from build123d import *

# Parameters (mm, degrees)
BOSS_EXTRUDE1_DEPTH = 40
CUT_EXTRUDE1_DEPTH  = 25
CUT_EXTRUDE2_DEPTH  = 15
SKETCH3_R           = 2.5
CUT_EXTRUDE3_DEPTH  = 16
SKETCH3_6_R         = 6
SKETCH3_6_R_2       = 2.5
BOSS_EXTRUDE2_DEPTH = 10
FILLET2_R           = 2


with BuildPart() as part:
    # Sketch1 → Boss-Extrude1 (new body)
    with BuildSketch(Plane.XY):
        with BuildLine():
            Line((0, 0), (-50, 0))
            Line((-50, 0), (-50, -12.5))
            Line((-50, -12.5), (-60, -12.5))
            Line((-60, -12.5), (-60, -50.5))
            Line((-60, -50.5), (-46, -50.5))
            Line((-46, -50.5), (-33.311690981, -44.583344336))
            ThreePointArc((-33.311690981, -44.583344336), (-24.66100943, -43.235991833), (-16.596266659, -46.643274342))
            Line((-16.596266659, -46.643274342), (-12, -50.5))
            Line((-12, -50.5), (0, -50.5))
            Line((0, -50.5), (0, 0))
        make_face()
    extrude(amount=-BOSS_EXTRUDE1_DEPTH)

    # Sketch2 → Cut-Extrude1 (cut)
    with BuildSketch(Plane.XY):
        with BuildLine():
            ThreePointArc((-53.849159388, -20.384615385), (-51.013665761, -16.887003184), (-50, -12.5))
            Line((-50, -12.5), (-60, -12.5))
            Line((-60, -12.5), (-60, -22.5))
            ThreePointArc((-60, -22.5), (-56.747781822, -21.956377579), (-53.849159388, -20.384615385))
        make_face()
        with BuildLine():
            Line((0, 0), (-30, 0))
            ThreePointArc((-30, 0), (-21.213203436, -21.213203436), (0, -30))
            Line((0, -30), (0, 0))
        make_face()
    extrude(amount=-CUT_EXTRUDE1_DEPTH, mode=Mode.SUBTRACT)

    # Sketch2_7 → Cut-Extrude2 (cut)
    with BuildSketch(Plane.XY):
        with BuildLine():
            ThreePointArc((-60, -33.5), (-52.756966211, -28.896831102), (-53.849159388, -20.384615385))
            ThreePointArc((-53.849159388, -20.384615385), (-56.747781822, -21.956377579), (-60, -22.5))
            Line((-60, -22.5), (-60, -33.5))
        make_face()
    extrude(amount=-CUT_EXTRUDE2_DEPTH, mode=Mode.SUBTRACT)

    # Sketch3 → Cut-Extrude3 (cut, through all)
    with BuildSketch(Plane.XY.offset(-25)):
        with Locations((-10, -10)):
            Circle(SKETCH3_R)
    extrude(amount=-CUT_EXTRUDE3_DEPTH, mode=Mode.SUBTRACT)

    # Sketch3_6 → Boss-Extrude2 (add)
    with BuildSketch(Plane.XY.offset(-25)):
        with Locations((-10, -10)):
            Circle(SKETCH3_6_R)
        with Locations((-10, -10)):
            Circle(SKETCH3_6_R_2, mode=Mode.SUBTRACT)
    extrude(amount=BOSS_EXTRUDE2_DEPTH)

    # Fillet2
    fillet2_edges = [part.edges().sort_by_distance(p)[0] for p in [
        (-16, -10, -25),
    ]]
    fillet(fillet2_edges, radius=FILLET2_R)


solid = part.part
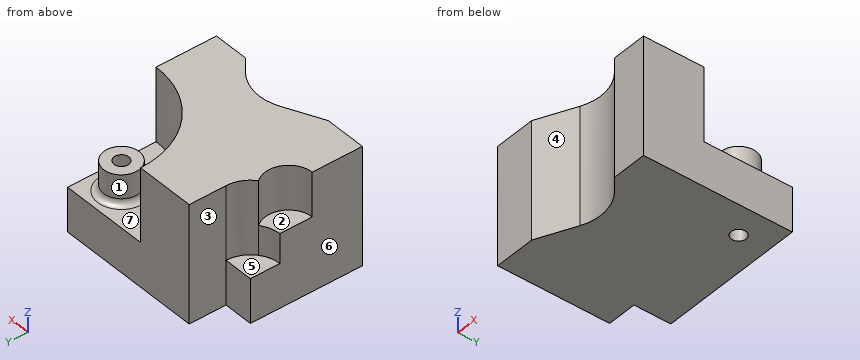
CAD build for the part. Positions are in the model's coordinates, mm. Face numbers are marked on the shaded views. A direction names the side the tool comes from. Round coordinates to 2 decimals unless told otherwise and drop trailing zeros. Order: outer loops, then holes, each group sorted by start corner. A loop starts at its lowest first (then second) coordinate and runs counter-clockwise, first axis right, second up. Notation, with made-up numbers: (68, 34.5) -> (101, 34.5) arc R28 cw to (101, 55.5) -> close; hole circle Ø8 at (69.25, 48.5). An arc over 180 degrees is marked (long way). Write item = value, one per line. Start each with the question number.
(1) Cut at A-A, the plane z = -8.5. List the corners of the cut face in (x, y).
(2) Cut at B-B, the plane x = -10. List the corners of the cut face in (y, z).
(3) Cut at D-D, the plane z = -28.5. List the corners of the cut face in (x, y), then the cut area to 3 significant figures.
(4) Pin check, flat tips, straight feed: P1, Ø3, axis at x = -57, z = -33.5, coming from the +Y side; P2, Ø4, axis at y = -28.5, z = -8, coming from the -X side (3 decimals); P3, Ø24, axis at x = -13, y = -12, coming from the +Z side; P4, Ø3, axis at x = -10, y = -10, coming from the +Z side. Stop position of each tip, or through.
(5) Cut at C-C, the plane y = -10. List the corners of the cut face in (x, z), then the cut area to 3 significant figures.
(6) Probe line 1 (Y direction, x = -10, z = -21.5); line 2 (Y direction, x = -10, z = -32); line 3 (Z direction, x = -22, y = -13). List the from-to ranges inside material, lowest first. Write a range as [from, to].
(7) Which spindle directions (+Z, -Z, +X, -X, +Y, -Y) get a long thin tool onto all of the face, cutting with end or side? Do the marked faces 1, 2, 3 and 4. Say none if no direction does.
(8) Pull direction X, two halves, no side cores. Call the marked faces 5, 6 and 7: released by +X, released by -X, zero draft, split by the parting line, or undercut.
Model answer:
q1.outline = (-60, -50.5) -> (-46, -50.5) -> (-33.31, -44.58) arc R16 cw to (-16.6, -46.64) -> (-12, -50.5) -> (0, -50.5) -> (0, -30) arc R30 cw to (-30, 0) -> (-50, 0) -> (-50, -12.5) arc R10 cw to (-53.85, -20.38) arc R8 cw to (-60, -33.5) -> close
q2.outline = (-50.5, -40) -> (-12.5, -40) -> (-12.5, -15) -> (-16, -15) -> (-16, -23) arc R2 cw to (-18, -25) -> (-28.28, -25) -> (-28.28, 0) -> (-50.5, 0) -> close; (-7.5, -40) -> (0, -40) -> (0, -25) -> (-2, -25) arc R2 cw to (-4, -23) -> (-4, -15) -> (-7.5, -15) -> close
q3.outline = (-60, -50.5) -> (-46, -50.5) -> (-33.31, -44.58) arc R16 cw to (-16.6, -46.64) -> (-12, -50.5) -> (0, -50.5) -> (0, 0) -> (-50, 0) -> (-50, -12.5) -> (-60, -12.5) -> close; hole circle Ø5 at (-10, -10)
q3.area = 2,730 mm2
q4.P1 = -12.5
q4.P2 = -53.755
q4.P3 = -15
q4.P4 = through
q5.outline = (-50, -40) -> (-12.5, -40) -> (-12.5, -15) -> (-16, -15) -> (-16, -23) arc R2 cw to (-18, -25) -> (-28.28, -25) -> (-28.28, 0) -> (-50, 0) -> close; (-7.5, -40) -> (0, -40) -> (0, -25) -> (-2, -25) arc R2 cw to (-4, -23) -> (-4, -15) -> (-7.5, -15) -> close
q5.area = 1,290 mm2
q6.line_1 = [-50.5, -28.28], [-16, -12.5], [-7.5, -4]
q6.line_2 = [-50.5, -12.5], [-7.5, 0]
q6.line_3 = [-40, -25]
q7.face_1 = +Z
q7.face_2 = +Z, -X
q7.face_3 = +Z, -Z, -X, +Y
q7.face_4 = +Z, -Z, -Y
q8.face_5 = zero draft
q8.face_6 = released by -X
q8.face_7 = undercut
